Autodesk Inventor part; units mm, degrees
ref_plane "YZ Plane" through (0, 0, 0) normal (1, 0, 0) x (0, 1, 0)
ref_plane "XZ Plane" through (0, 0, 0) normal (0, 1, 0) x (-1, 0, 0)
ref_plane "XY Plane" through (0, 0, 0) normal (0, 0, 1) x (1, 0, 0)
sketch "Sketch1" plane through (0, 0, 0) normal (0, 0, 1) x (1, 0, 0)
  circle A0 centre (0, 0) radius 3
  circle A1 centre (0, 0) radius 6
  dimension "d0" = 6
  dimension "d1" = 12
extrude "Extrusion1" add sketch "Sketch1" along normal blind 18.83
chamfer "Chamfer1" distance 1 angle 45 2 edges at (-6, 0, 18.83) (-6, 0, 0)
sketch "Sketch2" plane through (0, 0, 0) normal (1, 0, 0) x (0, 1, 0)
  line L0 (6.8077, 17.23) -> (5.6777, 17.23)
  line L1 (5.6777, 17.23) -> (5.6777, 16.1)
  line L2 (5.6777, 16.1) -> (6.8077, 16.1)
  line L3 (6.8077, 16.1) -> (6.8077, 17.23)
  line L4 (-5, 18.83) -> (5, 18.83)
  line L5 (6.8077, 1.6) -> (5.6777, 1.6)
  line L6 (5.6777, 1.6) -> (5.6777, 2.73)
  line L7 (5.6777, 2.73) -> (6.8077, 2.73)
  line L8 (6.8077, 2.73) -> (6.8077, 1.6)
  line L9 (5, 0) -> (-5, 0)
  line L10 (0, -3.766) -> (0, 22.596)
  point P0 (0, 0)
  dimension "d7" = 1.13
  dimension "d8" = 1.13
  dimension "d9" = 1.6
  dimension "d10" = 1.13
  dimension "d11" = 1.13
  dimension "d12" = 1.6
revolve "Revolution1" cut sketch "Sketch2" angle 360 about axis through (0, 0, -10) along (0, 0, 1)
properties part number "00_Igus_Drylin_6mm"
Can you work these out from the model? Positions are in its coordinate system, mm. A direction names the side the tool comes from. Coordinates: 2 decimals unless noted, no trailing zeros. Loops run counter-clockwise (first coordinate to the right, second up) from the corner with the lowest first, then second, coordinate; pieces in that order, holes last. Notation, with made-up numbers: (-31.5, 5) - (-23.5, 5) arc R32 ccw to (-23.5, 39) - close; hole circle Ø6 at (61, 46). An arc over 180 degrees is marked (long way). Use a Markdown table: item, result.
Item 1: Will these pins go through, and if not, where does the flat tip stop? pin 1 (3 mm diameter, centred on x = -4.5, z = 11.5, fed in from -Y); pin 2 (1.5 mm diameter, centred on y = 4, z = 13, fed in from -X).
Numbers:
| item | result |
|---|---|
| pin 1 | stops at y = -5.2 |
| pin 2 | stops at x = -5.04 |
Item 2: We'd pull the mould along X, two halves only. Please class faces 1 (the face through (5, 3, 16.1)), 2 (the face through (-3, 0, 9)), 3 (the face through (-5.63, -0.74, 2.17)): released by +X, released by -X, zero draft, split by the parting line, or undercut.
Numbers:
| item | result |
|---|---|
| face 1 | zero draft |
| face 2 | undercut |
| face 3 | split by the parting line |
Item 3: I want a section at D-D on z = 4. Please give me the cut outline in (x, y).
Numbers:
| item | result |
|---|---|
| outline | circle Ø12 at (0, 0); hole circle Ø6 at (0, 0) |
Item 4: I want a section at C-C on z = 16.75. Please give me the cut outline in (x, y).
Numbers:
| item | result |
|---|---|
| outline | circle Ø11.36 at (0, 0); hole circle Ø6 at (0, 0) |
Item 5: If I drill on probe 1 along Y at (x, z) = (0, 4.75); probe 2 along X at (y, z) = (-1, 16.75); probe 3 along Y at (x, z) = (1.25, 4.25), over which ranges is the centre line in solid material (lowest first)? Write a range as from..to.
Numbers:
| item | result |
|---|---|
| probe 1 | y = -6..-3, 3..6 |
| probe 2 | x = -5.59..-2.83, 2.83..5.59 |
| probe 3 | y = -5.87..-2.73, 2.73..5.87 |
Item 6: I want a section at A-A on y = 0. Please give me the cut outline in (x, z).
Numbers:
| item | result |
|---|---|
| outline | (-6, 1) - (-5, 0) - (-3, 0) - (-3, 18.83) - (-5, 18.83) - (-6, 17.83) - (-6, 17.23) - (-5.68, 17.23) - (-5.68, 16.1) - (-6, 16.1) - (-6, 2.73) - (-5.68, 2.73) - (-5.68, 1.6) - (-6, 1.6) - close; (3, 0) - (5, 0) - (6, 1) - (6, 1.6) - (5.68, 1.6) - (5.68, 2.73) - (6, 2.73) - (6, 16.1) - (5.68, 16.1) - (5.68, 17.23) - (6, 17.23) - (6, 17.83) - (5, 18.83) - (3, 18.83) - close |
Item 7: For faces 4 (the face through (3.3, 0.1, 18.83)), 5 (the face through (5, 3, 2.73)), which set-ups out of +Z, -Z, +X, -X, +Y, -Y let a thin tool reach every point of the face, with its end or its side?
Numbers:
| item | result |
|---|---|
| face 4 | +Z, +X, -X, +Y, -Y |
| face 5 | none |
